Drawing for the job (mm, zero at the part's lowest x, y, z). A direction names the side the tool comes from. Give positions to 0.01 mm unless a question says otherwise; leave off trailing zeros. Loops run counter-clockwise (first coordinate to the right, second up) from the corner with the lowest first, then second, coordinate; pieces in that order, holes last.
1) Flat gauge pins, fed straight in: P1, Ø12, axis at x = 20, y = 17, coming from the +Z side; P2, Ø1.5, axis at y = 26, z = 63, coming from the -X side; P3, Ø6, axis at y = 25, z = 67, coming from the +X side; P4, Ø0.6, axis at x = 25, z = 65, coming from the +Y side. Where does each tip first touch, or does it go through?
2) Two-plate mould, pull along X, no slides. Class the marked faces 1, 2, 3 and 4: +X half, -X half, draft (parallel to the pull), parting line (faces both ways), or undercut.
3) Wall check: line 1 (Y direction, x = 30.4, z = 62.8); line 2 (X direction, y = 51, z = 5); line 3 (Z direction, x = 49.5, y = 8). Give the ranges that are in metal, low to high.
4) 3-axis set-ups, long thin cutter, end or side, ignore diameter. For the marked faces 5, 6 and 7: which of +Z, -Z, +X, -X, +Y, -Y reach the whole face in a straight line?
5) Band-saw the part on C-C on x = 30. List the corners of the cut face in (y, z), then the cut area to 3 significant figures.
6) Band-saw the part on B-B on z = 62.8. List the corners of the cut face in (x, y).
7) Band-saw the part on D-D on y = 31.5. List the corners of the cut face in (x, z).
8) Band-saw the part on A-A on y = 20. List the corners of the cut face in (x, z), then the cut area to 3 significant figures.
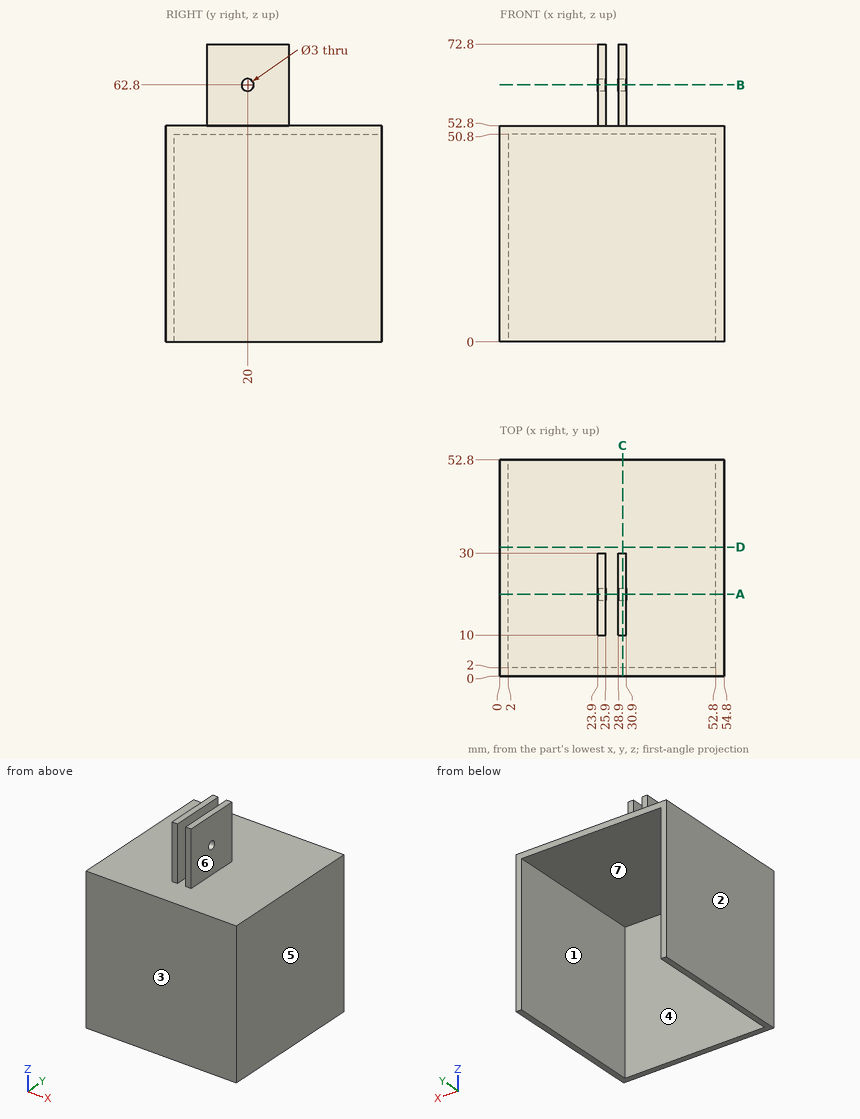
Findings below:
1. P1: stops at z = 72.8
1. P2: stops at x = 23.9
1. P3: stops at x = 30.9
1. P4: stops at y = 30
2. face 1: undercut
2. face 2: -X half
2. face 3: draft
2. face 4: undercut
3. line 1: y = 10 to 18.5, 21.5 to 30
3. line 2: x = 0 to 2, 52.8 to 54.8
3. line 3: z = 50.8 to 52.8
4. face 5: +Z, -Z, +X, +Y, -Y
4. face 6: +Z, +X, +Y, -Y
4. face 7: -Z, +Y
5. outline: (0, 0) - (2, 0) - (2, 50.8) - (52.8, 50.8) - (52.8, 52.8) - (30, 52.8) - (30, 72.8) - (10, 72.8) - (10, 52.8) - (0, 52.8) - close; hole circle Ø3 at (20, 62.8)
5. area: 600 mm2
6. outline: (23.9, 10) - (25.9, 10) - (25.9, 18.5) - (23.9, 18.5) - close; (23.9, 21.5) - (25.9, 21.5) - (25.9, 30) - (23.9, 30) - close; (28.9, 10) - (30.9, 10) - (30.9, 18.5) - (28.9, 18.5) - close; (28.9, 21.5) - (30.9, 21.5) - (30.9, 30) - (28.9, 30) - close
7. outline: (0, 0) - (2, 0) - (2, 50.8) - (52.8, 50.8) - (52.8, 0) - (54.8, 0) - (54.8, 52.8) - (0, 52.8) - close
8. outline: (0, 0) - (2, 0) - (2, 50.8) - (52.8, 50.8) - (52.8, 0) - (54.8, 0) - (54.8, 52.8) - (30.9, 52.8) - (30.9, 61.3) - (28.9, 61.3) - (28.9, 52.8) - (25.9, 52.8) - (25.9, 61.3) - (23.9, 61.3) - (23.9, 52.8) - (0, 52.8) - close; (23.9, 64.3) - (25.9, 64.3) - (25.9, 72.8) - (23.9, 72.8) - close; (28.9, 64.3) - (30.9, 64.3) - (30.9, 72.8) - (28.9, 72.8) - close
8. area: 381 mm2
